Read the model definition and answer for the solid it produces. Units are mm, in the model's axes. Face numbers are marked on the shaded views. Give positions to 0.01 mm unless a question says otherwise; leave off trailing zeros. Order: outer loops, then holes, each group sorted by start corner. A loop starts at its lowest first (then second) coordinate and runs counter-clockwise, first axis right, second up. Notation, with made-up numbers: (69.25, 52.5) - (102.25, 52.5) arc R19 ccw to (102.25, 58.5) - close; hole circle Ø5 at (-7, 85.5). An arc over 180 degrees is marked (long way). Write item = value, one per line.
```python
from build123d import *

# Parameters (mm, degrees)
F0_R     = 26
F0_R_2   = 12.5
F1_DEPTH = 18
F2_R     = 1
F3_R     = 1


with BuildPart() as f1:
    # F0 (on Front) → F1 (new body)
    with BuildSketch(Plane.XZ):
        Circle(F0_R)
        Circle(F0_R_2, mode=Mode.SUBTRACT)
    extrude(amount=F1_DEPTH)

    # F2
    f2_edges = [f1.edges().sort_by_distance(p)[0] for p in [
        (-26, -18, 0),
        (-26, 0, 0),
    ]]
    fillet(f2_edges, radius=F2_R)

    # F3
    f3_edges = [f1.edges().sort_by_distance(p)[0] for p in [
        (-12.5, -18, 0),
        (-12.5, 0, 0),
    ]]
    fillet(f3_edges, radius=F3_R)


solid = f1.part
```
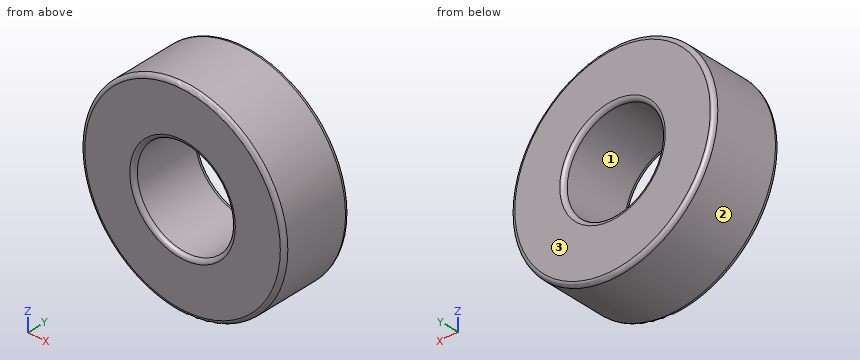
1. Section A-A (x = 0) is taken. Determine the outline of the cut face in (y, z).
Recorded:
outline = (-18, -25) arc R1 ccw to (-17, -26) - (-1, -26) arc R1 ccw to (0, -25) - (0, -13.5) arc R1 ccw to (-1, -12.5) - (-17, -12.5) arc R1 ccw to (-18, -13.5) - close; (-18, 13.5) arc R1 ccw to (-17, 12.5) - (-1, 12.5) arc R1 ccw to (0, 13.5) - (0, 25) arc R1 ccw to (-1, 26) - (-17, 26) arc R1 ccw to (-18, 25) - close
2. Section C-C (y = -4.5) is taken. Determine the outline of the cut face in (x, z), and give its area (3 significant figures).
Recorded:
outline = circle Ø52 at (0, 0); hole circle Ø25 at (0, 0)
area = 1,630 mm^2
3. Straight lines are drawn through the part: L1, parallel to Z at x = 0, y = -5; L2, parallel to Z at x = 3.5, y = -16.5; L3, parallel to X at y = -13.25, z = 2. For each, find the intervals that lie inside material, in ascending order. Write a range as [from, to].
Recorded:
L1 = [-26, -12.5], [12.5, 26]
L2 = [-25.76, -12], [12, 25.76]
L3 = [-25.92, -12.34], [12.34, 25.92]
4. Determine the mould class of the marked faces 1, 2 and 3 for opening direction Z: +Z half, -Z half, draft (parallel to the pull), parting line (faces both ways), or undercut.
Recorded:
face_1 = undercut
face_2 = parting line
face_3 = draft
5. Section B-B (z = 0) is taken. Determine the outline of the cut face in (x, y).
Recorded:
outline = (-26, -17) arc R1 ccw to (-25, -18) - (-13.5, -18) arc R1 ccw to (-12.5, -17) - (-12.5, -1) arc R1 ccw to (-13.5, 0) - (-25, 0) arc R1 ccw to (-26, -1) - close; (12.5, -17) arc R1 ccw to (13.5, -18) - (25, -18) arc R1 ccw to (26, -17) - (26, -1) arc R1 ccw to (25, 0) - (13.5, 0) arc R1 ccw to (12.5, -1) - close
6. Flat-ended cylindrical pins translate along their axes: pin 1 (2 mm diameter, centred on y = -10.5, z = -12, fed in from +X); pin 2 (1.5 mm diameter, centred on x = -3, z = 11, fed in from -Y); pin 3 (6 mm diameter, centred on x = -7.5, y = -14, fed in from -Z); pin 4 (1 mm diameter, centred on x = 6.5, y = -9.5, fed in from +Z). Find the tip coordinate at first contact, or state that the pin passes through.
Recorded:
pin_1 = 23.56
pin_2 = through
pin_3 = -25.61
pin_4 = 25.3
